```python
from build123d import *

# Parameters (mm, degrees)
SKETCH_2_R      = 40.75
SKETCH_2_R_2    = 1.5
EXTRUDE_1_DEPTH = 3
FILLET_1_R      = 1
FILLET_2_R      = 2


with BuildPart() as part:
    # 草图2 → 凸台-拉伸1 (new body)
    with BuildSketch(Plane.XY):
        with BuildLine():
            Line((10, 58.653644388), (10, 43.839202169))
            ThreePointArc((10, 43.839202169), (0, 43), (-10, 43.839202169))
            Line((-10, 43.839202169), (-10, 58.653644388))
            ThreePointArc((-10, 58.653644388), (-16.763087132, 57.08983193), (-23.29801892, 54.748993729))
            Line((-23.29801892, 54.748993729), (-15.288726769, 42.286291876))
            ThreePointArc((-15.288726769, 42.286291876), (-23.247555151, 36.173901912), (-32.113797426, 31.473475527))
            Line((-32.113797426, 31.473475527), (-40.123089577, 43.93617738))
            ThreePointArc((-40.123089577, 43.93617738), (-44.967099674, 38.96421367), (-49.199081449, 33.4619244))
            Line((-49.199081449, 33.4619244), (-35.723390814, 27.307782693))
            ThreePointArc((-35.723390814, 27.307782693), (-39.1141758, 17.862845559), (-44.031691074, 9.115142785))
            Line((-44.031691074, 9.115142785), (-57.50738171, 15.269284493))
            ThreePointArc((-57.50738171, 15.269284493), (-58.894375792, 8.467732877), (-59.479783242, 1.550930504))
            Line((-59.479783242, 1.550930504), (-44.816130685, 3.659245452))
            ThreePointArc((-44.816130685, 3.659245452), (-42.562322001, -6.119538046), (-41.969833919, -16.137183386))
            Line((-41.969833919, -16.137183386), (-56.633486477, -18.245498334))
            ThreePointArc((-56.633486477, -18.245498334), (-54.123103724, -24.717193274), (-50.87607412, -30.852472869))
            Line((-50.87607412, -30.852472869), (-39.680065719, -21.151076364))
            ThreePointArc((-39.680065719, -21.151076364), (-32.497231697, -28.15901156), (-26.58285104, -36.266067852))
            Line((-26.58285104, -36.266067852), (-37.778859441, -45.967464356))
            ThreePointArc((-37.778859441, -45.967464356), (-32.168128639, -50.054585203), (-26.119570938, -53.460434099))
            Line((-26.119570938, -53.460434099), (-21.945860253, -39.246080882))
            ThreePointArc((-21.945860253, -39.246080882), (-12.114499944, -41.258197865), (-2.756000781, -44.880732018))
            Line((-2.756000781, -44.880732018), (-6.929711465, -59.095085236))
            ThreePointArc((-6.929711465, -59.095085236), (0, -59.5), (6.929711465, -59.095085236))
            Line((6.929711465, -59.095085236), (2.756000781, -44.880732018))
            ThreePointArc((2.756000781, -44.880732018), (12.114499944, -41.258197865), (21.945860253, -39.246080882))
            Line((21.945860253, -39.246080882), (26.119570938, -53.460434099))
            ThreePointArc((26.119570938, -53.460434099), (32.168128639, -50.054585203), (37.778859441, -45.967464356))
            Line((37.778859441, -45.967464356), (26.58285104, -36.266067852))
            ThreePointArc((26.58285104, -36.266067852), (32.497231697, -28.15901156), (39.680065719, -21.151076364))
            Line((39.680065719, -21.151076364), (50.87607412, -30.852472869))
            ThreePointArc((50.87607412, -30.852472869), (54.123103724, -24.717193274), (56.633486477, -18.245498334))
            Line((56.633486477, -18.245498334), (41.969833919, -16.137183386))
            ThreePointArc((41.969833919, -16.137183386), (42.562322001, -6.119538046), (44.816130685, 3.659245452))
            Line((44.816130685, 3.659245452), (59.479783242, 1.550930504))
            ThreePointArc((59.479783242, 1.550930504), (58.894375792, 8.467732877), (57.50738171, 15.269284493))
            Line((57.50738171, 15.269284493), (44.031691074, 9.115142785))
            ThreePointArc((44.031691074, 9.115142785), (39.1141758, 17.862845559), (35.723390814, 27.307782693))
            Line((35.723390814, 27.307782693), (49.199081449, 33.4619244))
            ThreePointArc((49.199081449, 33.4619244), (44.967099674, 38.96421367), (40.123089577, 43.93617738))
            Line((40.123089577, 43.93617738), (32.113797426, 31.473475527))
            ThreePointArc((32.113797426, 31.473475527), (23.247555151, 36.173901912), (15.288726769, 42.286291876))
            Line((15.288726769, 42.286291876), (23.29801892, 54.748993729))
            ThreePointArc((23.29801892, 54.748993729), (16.763087132, 57.08983193), (10, 58.653644388))
        make_face()
        Circle(SKETCH_2_R, mode=Mode.SUBTRACT)
        with Locations((0, -51.5)):
            Circle(SKETCH_2_R_2, mode=Mode.SUBTRACT)
        with Locations((-27.843002099, -43.324556941)):
            Circle(SKETCH_2_R_2, mode=Mode.SUBTRACT)
        with Locations((-46.846047761, -21.39387317)):
            Circle(SKETCH_2_R_2, mode=Mode.SUBTRACT)
        with Locations((-50.975804257, 7.329214171)):
            Circle(SKETCH_2_R_2, mode=Mode.SUBTRACT)
        with Locations((-38.921103079, 33.725327798)):
            Circle(SKETCH_2_R_2, mode=Mode.SUBTRACT)
        with Locations((-14.509226677, 49.413888141)):
            Circle(SKETCH_2_R_2, mode=Mode.SUBTRACT)
        with Locations((14.509226677, 49.413888141)):
            Circle(SKETCH_2_R_2, mode=Mode.SUBTRACT)
        with Locations((38.921103079, 33.725327798)):
            Circle(SKETCH_2_R_2, mode=Mode.SUBTRACT)
        with Locations((50.975804257, 7.329214171)):
            Circle(SKETCH_2_R_2, mode=Mode.SUBTRACT)
        with Locations((46.846047761, -21.39387317)):
            Circle(SKETCH_2_R_2, mode=Mode.SUBTRACT)
        with Locations((27.843002099, -43.324556941)):
            Circle(SKETCH_2_R_2, mode=Mode.SUBTRACT)
    extrude(amount=EXTRUDE_1_DEPTH)

    # 圆角1
    fillet_1_edges = [part.edges().sort_by_distance(p)[0] for p in [
        (15.288726769, 42.286291876, 1.5),
        (32.113797426, 31.473475527, 1.5),
        (35.723390814, 27.307782693, 1.5),
        (44.031691074, 9.115142785, 1.5),
        (44.816130685, 3.659245452, 1.5),
        (41.969833919, -16.137183386, 1.5),
        (39.680065719, -21.151076364, 1.5),
        (26.58285104, -36.266067852, 1.5),
        (21.945860253, -39.246080882, 1.5),
        (2.756000781, -44.880732018, 1.5),
        (-2.756000781, -44.880732018, 1.5),
        (-21.945860253, -39.246080882, 1.5),
        (-26.58285104, -36.266067852, 1.5),
        (-39.680065719, -21.151076364, 1.5),
        (-41.969833919, -16.137183386, 1.5),
        (-44.816130685, 3.659245452, 1.5),
        (-44.031691074, 9.115142785, 1.5),
        (-35.723390814, 27.307782693, 1.5),
        (-32.113797426, 31.473475527, 1.5),
        (-15.288726769, 42.286291876, 1.5),
        (-10, 43.839202169, 1.5),
        (10, 43.839202169, 1.5),
    ]]
    fillet(fillet_1_edges, radius=FILLET_1_R)

    # 圆角2
    fillet_2_edges = [part.edges().sort_by_distance(p)[0] for p in [
        (23.29801892, 54.748993729, 1.5),
        (40.123089577, 43.93617738, 1.5),
        (49.199081449, 33.4619244, 1.5),
        (57.50738171, 15.269284493, 1.5),
        (59.479783242, 1.550930504, 1.5),
        (56.633486477, -18.245498334, 1.5),
        (50.87607412, -30.852472869, 1.5),
        (37.778859441, -45.967464356, 1.5),
        (26.119570938, -53.460434099, 1.5),
        (6.929711465, -59.095085236, 1.5),
        (-6.929711465, -59.095085236, 1.5),
        (-26.119570938, -53.460434099, 1.5),
        (-37.778859441, -45.967464356, 1.5),
        (-50.87607412, -30.852472869, 1.5),
        (-56.633486477, -18.245498334, 1.5),
        (-59.479783242, 1.550930504, 1.5),
        (-57.50738171, 15.269284493, 1.5),
        (-49.199081449, 33.4619244, 1.5),
        (-40.123089577, 43.93617738, 1.5),
        (-23.29801892, 54.748993729, 1.5),
        (-10, 58.653644388, 1.5),
        (10, 58.653644388, 1.5),
    ]]
    fillet(fillet_2_edges, radius=FILLET_2_R)


solid = part.part
```
Model file for the job. Use its own axes, mm. A direction names the side the tool comes from. Coordinates: 2 decimals unless noted, no trailing zeros. Order: outer loops, then holes, each group sorted by start corner. A loop starts at its lowest first (then second) coordinate and runs counter-clockwise, first axis right, second up. Notation, with made-up numbers: (-14, -34) -> (-8, -34) arc R15 cw to (-8, -18) -> close; hole circle Ø1 at (30, 4). An arc over 180 degrees is marked (long way). Answer as a JSON object with one key per item and string values. Group by question number.
1) Cut at D-D, the plane z = 2.5. Count the separate pieces of the cut face and the enclosed holes in it, then the cut area to 3 significant figures.
2) Cut at B-B, the plane y = 30. Write the cut outline in (x, z), then the cut area to 3 significant figures.
3) Cut at C-C, the plane y = 0. Write the cut outline in (x, z).
4) Which spindle directions (+Z, -Z, +X, -X, +Y, -Y) get a long thin tool onto all of the face, cutting with end or side? Do faces 1 (the face through (5.99, -58.45, 1.52)), 2 (the face through (32.41, -28.26, 1.48)), 3 (the face through (-23.835, -45.678, 1.479)). Say none if no direction does.
5) Pull direction Y, two halves, no side cores. Call faces 4 (the face through (-36.64, -45.94, 1.52)), 5 (the face through (-44.7, -25.5, 1.5)), 6 (the face through (45.008, 38.917, 1.479)): +Y half, -Y half, draft (parallel to the pull), parting line (faces both ways), or undercut.
6) Cut at A-A, the plane x = 0. Write the cut outline in (y, z).
7) Flat gauge pins, fed straight in: pin 1 (1 mm diameter, centred on x = -36, z = 2.5, fed in from +Y); pin 2 (2.5 mm diameter, centred on x = 14.51, y = 49.41, fed in from -Z); pin 3 (3.5 mm diameter, centred on x = -27.84, y = -43.32, fed in from -Z); pin 4 (1 mm diameter, centred on y = 45.5, z = 0.5, fed in from -X). Where does each tip first touch, or does it go through?
8) Drill centre lines: L1, parallel to Y at x = 48, z = 1.1; L2, parallel to Y at x = -30.5, z = 1.5; L3, parallel to Y at x = 15.5, z = 2.35. Where is each one in solid material? Low to high.
Check values:
{
 "1": {"separate pieces": "1", "enclosed holes": "12", "area": "2,290 mm²"},
 "2": {"outline": "(-41.62, 0) -> (-27.58, 0) -> (-27.58, 3) -> (-41.62, 3) -> close; (27.58, 0) -> (41.62, 0) -> (41.62, 3) -> (27.58, 3) -> close", "area": "84.2 mm²"},
 "3": {"outline": "(-43.77, 0) -> (-40.75, 0) -> (-40.75, 3) -> (-43.77, 3) -> close; (40.75, 0) -> (43.77, 0) -> (43.77, 3) -> (40.75, 3) -> close"},
 "4": {"face 1": "+Z, -Z, +X", "face 2": "+Z, -Z", "face 3": "+Z, -Z, -Y"},
 "5": {"face 4": "undercut", "face 5": "-Y half", "face 6": "+Y half"},
 "6": {"outline": "(-59.5, 0) -> (-53, 0) -> (-53, 3) -> (-59.5, 3) -> close; (-50, 0) -> (-40.75, 0) -> (-40.75, 3) -> (-50, 3) -> close; (40.75, 0) -> (43, 0) -> (43, 3) -> (40.75, 3) -> close"},
 "7": {"pin 1": "stops at y = 38.3", "pin 2": "passes through", "pin 3": "stops at z = 0", "pin 4": "stops at x = -17.68"},
 "8": {"L1": "y = -28.36 to -22.35, -20.44 to -17, 3.2 to 10.93, 33.48 to 35.08", "L2": "y = -51.09 to -39.66, -30.59 to -27.02, 27.02 to 32.19", "L3": "y = -40.37 to -37.69, 37.69 to 48.29, 50.54 to 57.45"}
}
